Build history of the part. All positions in model axes, mm. A direction names the side the tool comes from. Round coordinates to 2 decimals unless told otherwise and drop trailing zeros. Write each loop counter-clockwise with the first axis right and the second up, starting at its lowest first coordinate (ties: lowest second). Pieces come first, ordered by that corner, then holes. Notation, with made-up numbers: (73.5, 42.25) -> (132.5, 42.25) arc R18 cw to (132.5, 52.25) -> close; hole circle Ø3 at (19, 82). An arc over 180 degrees is marked (long way). Answer in a Markdown table with one row per item.
```python
from build123d import *

# Parameters (mm, degrees)
F1_DEPTH = 82.55
F2_W     = 82.55
F2_H     = 154.17393
F3_DEPTH = 20.32
F4_W     = 25.331251
F4_H     = 78.070102
F4_W_2   = 27.407586
F4_H_2   = 78.070093
F5_DEPTH = 76.2
F6_W     = 25.331251
F6_H     = 70.189761
F6_W_2   = 27.407586
F7_DEPTH = 3.81


with BuildPart() as f1:
    # F0 (on Right) → F1 (new body)
    with BuildSketch(Plane.YZ):
        Polygon((-5.292215, 52.064744), (-70.189761, -26.107301), (62.555218, -26.107301), (62.555218, 52.064744), align=None)
    extrude(amount=-F1_DEPTH)

    # F2 (on face) → F3 (join)
    with BuildSketch(Plane(origin=(0, 62.555218, 0), x_dir=(-1, 0, 0), z_dir=(0, 1, 0))):
        with Locations((41.275, 50.979664)):
            Rectangle(F2_W, F2_H)
    extrude(amount=F3_DEPTH)

    # F4 (on Front) → F5 (cut)
    with BuildSketch(Plane.XZ):
        with Locations((-59.212166, 12.739294)):
            Rectangle(F4_W, F4_H)
        with Locations((-22.461083, 12.739295)):
            Rectangle(F4_W_2, F4_H_2)
    extrude(amount=F5_DEPTH, mode=Mode.SUBTRACT)

    # F6 (on face) → F7 (join)
    with BuildSketch(Plane(origin=(0, 0, -26.107301), x_dir=(1, 0, 0), z_dir=(0, 0, -1))):
        with Locations((-59.212166, 35.09488)):
            Rectangle(F6_W, F6_H)
        with Locations((-22.461083, 35.09488)):
            Rectangle(F6_W_2, F6_H)
    extrude(amount=-F7_DEPTH)


solid = f1.part
```
Q1. Two-plate mould, pull along Z, no slides. Class faces 1 (the flat face through (-59, -70.19, -24)), 2 (the flat face through (-59, 0, 15)), 3 (the flat face through (-42, 5, -26.107)): released by +Z, released by -Z, zero draft, split by the parting line, or undercut.
A:
| item | result |
|---|---|
| face 1 | zero draft |
| face 2 | undercut |
| face 3 | released by -Z |
Q2. Saw through at B-B on y = -38. Write the cut outline in (x, z).
A:
| item | result |
|---|---|
| outline | (-82.55, -26.11) -> (0, -26.11) -> (0, 12.67) -> (-8.76, 12.67) -> (-8.76, -22.3) -> (-36.16, -22.3) -> (-36.16, 12.67) -> (-46.55, 12.67) -> (-46.55, -22.3) -> (-71.88, -22.3) -> (-71.88, 12.67) -> (-82.55, 12.67) -> close |
Q3. Saw through at A-A on x = -24. Write the cut outline in (y, z), plus the area to 3 significant figures.
A:
| item | result |
|---|---|
| outline | (-70.19, -26.11) -> (82.88, -26.11) -> (82.88, 128.07) -> (62.56, 128.07) -> (62.56, 52.06) -> (-5.29, 52.06) -> (-5.53, 51.77) -> (0, 51.77) -> (0, -22.3) -> (-70.19, -22.3) -> close |
| area | 8,290 mm² |
Q4. Saw through at D-D on x = -74.5. Write the cut outline in (y, z).
A:
| item | result |
|---|---|
| outline | (-70.19, -26.11) -> (82.88, -26.11) -> (82.88, 128.07) -> (62.56, 128.07) -> (62.56, 52.06) -> (-5.29, 52.06) -> close |
Q5. Wall check: line 1 (X direction, y = -25, z = 3.5); line 2 (Y direction, x = -18, z = 66); line 3 (Z direction, x = -51, y = 31.5). Give the ranges that are in metal, low to high. Write a range as [from, to].
A:
| item | result |
|---|---|
| line 1 | [-82.55, -71.88], [-46.55, -36.16], [-8.76, 0] |
| line 2 | [62.56, 82.88] |
| line 3 | [-26.11, 52.06] |
Q6. Which spindle directions (+Z, -Z, +X, -X, +Y, -Y) get a long thin tool onto all of the face, cutting with end or side? Do faces 4 (the flat face through (-36.165, -26, 6)), 5 (the flat face through (-41, 62.555, 91)), 6 (the flat face through (-23, -70.19, -24)). Say none if no direction does.
A:
| item | result |
|---|---|
| face 4 | -Y |
| face 5 | +Z, +X, -X, -Y |
| face 6 | +Z, -Z, +X, -X, -Y |
Q7. Drop flat-ended pins along their axis: P1, Ø5, axis at x = -29, z = 88, coming from the -Y side; P2, Ø22, axis at x = -21.5, z = 21.5, coming from the -Y side; P3, Ø20.5, axis at x = -31, y = 17.5, coming from the +Z side. Give the stop position or say it passes through.
A:
| item | result |
|---|---|
| P1 | y = 62.56 |
| P2 | y = 0 |
| P3 | z = 52.06 |
Q8. Saw through at C-C on z = -11. Write the cut outline in (x, y), plus the area to 3 significant figures.
A:
| item | result |
|---|---|
| outline | (-82.55, -57.65) -> (-71.88, -57.65) -> (-71.88, 0) -> (-46.55, 0) -> (-46.55, -57.65) -> (-36.16, -57.65) -> (-36.16, 0) -> (-8.76, 0) -> (-8.76, -57.65) -> (0, -57.65) -> (0, 82.88) -> (-82.55, 82.88) -> close |
| area | 8,560 mm² |
